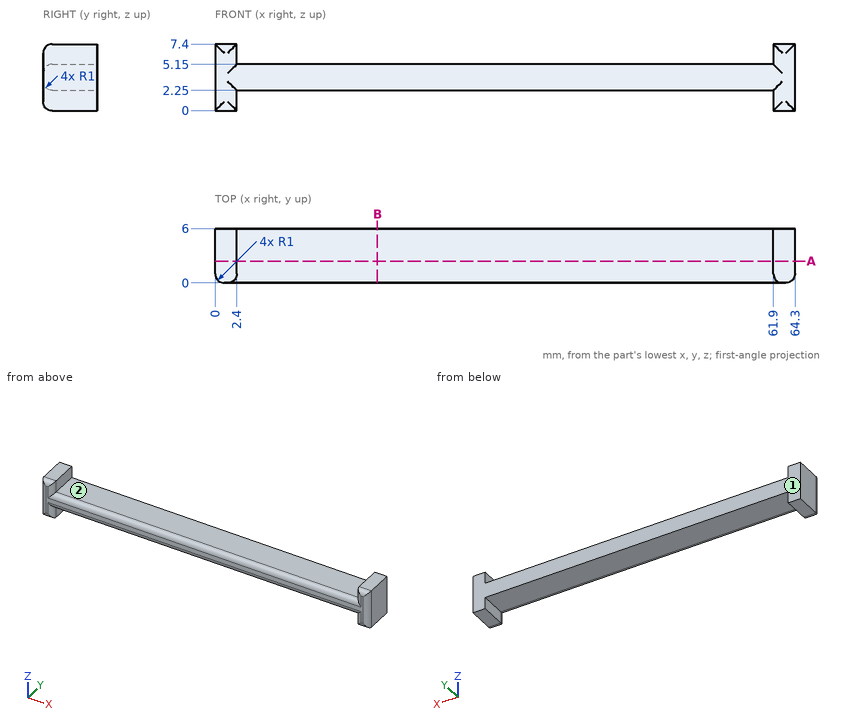
Can you work these out from the drawing? Everything is in mm from the part's minimum corner. Round coordinates to 2 decimals unless told otherwise and drop trailing zeros. Loops run counter-clockwise (first coordinate to the right, second up) from the corner with the lowest first, then second, coordinate; pieces in that order, holes last. Notation, with made-up numbers: (88, 55.5) -> (99, 55.5) arc R25 cw to (99, 83.5) -> close; hole circle Ø3 at (-25, 35). An arc over 180 degrees is marked (long way). Put each result on its own line as item: value.
Q1. Please list where these lines run through material, in increasing order: line 1 (X direction, y = 3.7, z = 2); line 2 (Z direction, x = 33, y = 4.15). Write a range as from..to.
Checks:
line 1: 0..2.4, 61.9..64.3
line 2: 2.25..5.15
Q2. Thinking about a two-plate mould opening in X: for the marked faces 1 and 2, which applies, pulls with the +X half, pulls with the -X half, needs draft (parallel to the pull), parting line crosses it, or undercut?
Checks:
face 1: needs draft
face 2: undercut
Q3. For pin 1 Ø0.7 at (y, z) = (3.5, 1.5) entering from -X; pin 2 Ø3 at (x, y) = (47.5, 5) entering from +Z; pin 3 Ø1.5 at (x, y) = (30, 3) entering from -Z, each with a flat end and sliding along its axis, tell me the tip position at first contact or that it passes through.
Checks:
pin 1: x = 0
pin 2: z = 5.15
pin 3: z = 2.25
Q4. I want a section at A-A on y = 2.4. Write out the boundary of the cut face in (x, z).
Checks:
outline: (0, 0) -> (2.4, 0) -> (2.4, 2.25) -> (61.9, 2.25) -> (61.9, 0) -> (64.3, 0) -> (64.3, 7.4) -> (61.9, 7.4) -> (61.9, 5.15) -> (2.4, 5.15) -> (2.4, 7.4) -> (0, 7.4) -> close
Q5. I want a section at B-B on x = 18. Write out the boundary of the cut face in (y, z).
Checks:
outline: (0, 3.25) arc R1 ccw to (1, 2.25) -> (6, 2.25) -> (6, 5.15) -> (1, 5.15) arc R1 ccw to (0, 4.15) -> close
